Could you check a few things on this model? Use its own coordinates, in mm. A direction names the side the tool comes from. Round coordinates to 2 decimals unless told otherwise and drop trailing zeros. Loops run counter-clockwise (first coordinate to the right, second up) from the corner with the lowest first, then second, coordinate; pieces in that order, holes last. Notation, with made-up numbers: M 51,84 L 106,84 A18 cw 106,99 Z; hole C 58,38.25 d8. An arc over 180 degrees is marked long. One line per item, written item: value. Start each with the question number.
Q1. I'm going to push flat-ended pins straight in: pin 1 Ø2.5 at (x, z) = (88.5, 4) entering from -Y; pin 2 Ø6.5 at (x, y) = (-56, 0) entering from +Z; pin 3 Ø1.3 at (x, y) = (-0.5, -99.5) entering from +Z. Where does each tip first touch, or does it pass through?
Q2. Please list where these lines run through material, in increasing order: line 1 along Y through (x, z) = (0, 7.4); line 2 along Y through (x, z) = (0, 2.3); line 3 along Y through (x, z) = (99, 5.9).
Q3. Imagine slicing it at C-C (z = 6.5). Give the number of separate pieces and of enclosed holes in the cut face, then the cut area to 3 significant figures.
Q4. Which directions (+Z, -Z, +X, -X, +Y, -Y) give clear straight access to the entire face, cutting with the end or side of a thin tool? Please do faces 1 (the face through (-91, 5, 4)), 2 (the face through (5, -91, 4)), 3 (the face through (-5, -91, 4)).
Q5. Imagine slicing it at D-D (y = 73). Please give me the cut outline in (x, z).
Q6. Imagine slicing it at B-B (y = 47.5). Please give me the cut outline in (x, z).
Q7. Imagine slicing it at A-A (x = 31). Please give me the cut outline in (y, z).
from build123d import *

# Parameters (mm, degrees)
CROQUIS1_R              = 60.25
CROQUIS1_R_2            = 2
CROQUIS1_R_3            = 53.25
SALIENTE_EXTRUIR1_DEPTH = 5
CROQUIS1_2_R            = 63.25
CROQUIS1_2_R_2          = 60.25
EXTRUIR_L_MINA1_DEPTH   = 8
CROQUIS2_W              = 10
CROQUIS2_H              = 40.947938178
CROQUIS2_R              = 1.25
CROQUIS2_W_2            = 40.947938178
CROQUIS2_H_2            = 10
SALIENTE_EXTRUIR2_DEPTH = 8
REDONDEO1_R             = 25
CROQUIS3_R              = 2.15
CORTAR_EXTRUIR1_DEPTH   = 5
REDONDEO2_R             = 5


with BuildPart() as part:
    # Croquis1 → Saliente-Extruir1 (new body)
    with BuildSketch(Plane.XY):
        Circle(CROQUIS1_R)
        with Locations((0, 56)):
            Circle(CROQUIS1_R_2, mode=Mode.SUBTRACT)
        Circle(CROQUIS1_R_3, mode=Mode.SUBTRACT)
        with Locations((56, 0)):
            Circle(CROQUIS1_R_2, mode=Mode.SUBTRACT)
        with Locations((0, -56)):
            Circle(CROQUIS1_R_2, mode=Mode.SUBTRACT)
        with Locations((-56, 0)):
            Circle(CROQUIS1_R_2, mode=Mode.SUBTRACT)
    extrude(amount=SALIENTE_EXTRUIR1_DEPTH)

    # Croquis1<2> → Extruir-Lámina1 (add)
    with BuildSketch(Plane.XY):
        Circle(CROQUIS1_2_R)
        Circle(CROQUIS1_2_R_2, mode=Mode.SUBTRACT)
    extrude(amount=EXTRUIR_L_MINA1_DEPTH)

    # Croquis2 → Saliente-Extruir2 (add)
    # profile 1 of 4: a face of its own
    with BuildSketch(Plane.XY):
        with Locations((0, 83.526030911)):
            Rectangle(CROQUIS2_W, CROQUIS2_H)
        with Locations((0, 99)):
            Circle(CROQUIS2_R, mode=Mode.SUBTRACT)
    # profile 2 of 4: a face of its own
    with BuildSketch(Plane.XY):
        with Locations((83.526030911, 0)):
            Rectangle(CROQUIS2_W_2, CROQUIS2_H_2)
        with Locations((99, 0)):
            Circle(CROQUIS2_R, mode=Mode.SUBTRACT)
    # profile 3 of 4: a face of its own
    with BuildSketch(Plane.XY):
        with Locations((0, -83.526030911)):
            Rectangle(CROQUIS2_W, CROQUIS2_H)
        with Locations((0, -99)):
            Circle(CROQUIS2_R, mode=Mode.SUBTRACT)
    # profile 4 of 4: a face of its own
    with BuildSketch(Plane.XY):
        with Locations((-83.526030911, 0)):
            Rectangle(CROQUIS2_W_2, CROQUIS2_H_2)
        with Locations((-99, 0)):
            Circle(CROQUIS2_R, mode=Mode.SUBTRACT)
    extrude(amount=SALIENTE_EXTRUIR2_DEPTH)

    # Redondeo1
    redondeo1_edges = [part.edges().sort_by_distance(p)[0] for p in [
        (-5, 63.052061822, 4),
        (5, 63.052061822, 4),
        (63.052061822, 5, 4),
        (63.052061822, -5, 4),
        (5, -63.052061822, 4),
        (-5, -63.052061822, 4),
        (-63.052061822, -5, 4),
        (-63.052061822, 5, 4),
    ]]
    fillet(redondeo1_edges, radius=REDONDEO1_R)

    # Croquis3 → Cortar-Extruir1 (cut)
    with BuildSketch(Plane.XY.offset(8)):
        with Locations((0, 99)):
            Circle(CROQUIS3_R)
        with Locations((99, 0)):
            Circle(CROQUIS3_R)
        with Locations((0, -99)):
            Circle(CROQUIS3_R)
        with Locations((-99, 0)):
            Circle(CROQUIS3_R)
    extrude(amount=-CORTAR_EXTRUIR1_DEPTH, mode=Mode.SUBTRACT)

    # Redondeo2
    redondeo2_edges = [part.edges().sort_by_distance(p)[0] for p in [
        (-104, -5, 4),
        (-104, 5, 4),
        (-5, -104, 4),
        (5, -104, 4),
        (104, -5, 4),
        (104, 5, 4),
        (5, 104, 4),
        (-5, 104, 4),
    ]]
    fillet(redondeo2_edges, radius=REDONDEO2_R - 0.0001)  # a hair under: the kernel refuses the full size


solid = part.part
Report:
1. pin 1: stops at y = -5
1. pin 2: stops at z = 5
1. pin 3: stops at z = 3
2. line 1: y = -104 to -101.15, -96.85 to -60.25, 60.25 to 96.85, 101.15 to 104
2. line 2: y = -104 to -100.25, -97.75 to -58, -54 to -53.25, 53.25 to 54, 58 to 97.75, 100.25 to 104
2. line 3: y = -5 to -2.15, 2.15 to 5
3. separate pieces: 1
3. enclosed holes: 5
3. area: 3,250 mm²
4. face 1: +Z, -Z, -X, +Y
4. face 2: +Z, -Z, +X, -Y
4. face 3: +Z, -Z, -X, -Y
5. outline: M -7.08,0 L 7.08,0 L 7.08,8 L -7.08,8 Z
6. outline: M -41.76,0 L -24.07,0 L -24.07,5 L -37.06,5 L -37.06,8 L -41.76,8 Z; M 24.07,0 L 41.76,0 L 41.76,8 L 37.06,8 L 37.06,5 L 24.07,5 Z
7. outline: M -55.13,0 L -43.3,0 L -43.3,5 L -51.66,5 L -51.66,8 L -55.13,8 Z; M 43.3,0 L 55.13,0 L 55.13,8 L 51.66,8 L 51.66,5 L 43.3,5 Z
